Part model, mm, in its own coordinate system. Round coordinates to 2 decimals unless told otherwise and drop trailing zeros. Loops run counter-clockwise (first coordinate to the right, second up) from the corner with the lowest first, then second, coordinate; pieces in that order, holes last.
1) Drop flat-ended pins along their axis: P1, Ø3, axis at y = 1, z = -128.5, coming from the +X side; P2, Ø1.5, axis at x = 81.5, y = 2.5, coming from the +Z side; P3, Ø1, axis at x = -37, y = 4, coming from the -Z side. Give the stop position or say it passes through.
2) Band-saw the part on A-A, the plane x = 31. Write the cut outline in (y, z).
3) Probe line 1 (X direction, y = 3, z = -80); line 2 (Z direction, x = -93, y = 2.85); line 3 (Z direction, x = 26.5, y = 0.7). List the from-to ranges inside material, lowest first.
4) Band-saw the part on B-B, the plane y = 3.45. State how many separate pieces and enclosed holes the cut face has, then the cut area to 3 significant figures.
5) Band-saw the part on C-C, the plane x = -88.5. Write the cut outline in (y, z), then the cut area to 4 significant figures.
from build123d import *

# Parameters (mm, degrees)
SKETCH_1_W           = 213
SKETCH_1_H           = 190
EXTRUDE_1_DEPTH      = 5
SKETCH_2_R           = 2
SKETCH_2_R_2         = 6
CUT_EXTRUDE_1_DEPTH  = 143.801435567
SKETCH_3_W           = 213
SKETCH_3_H           = 5.445794932
CUT_EXTRUDE_2_DEPTH  = 143.801435567
SKETCH_4_W           = 28
SKETCH_4_H           = 35
CUT_EXTRUDE_3_DEPTH  = 143.801435567
FILLET_1_R           = 5
SKETCH_5_W           = 42
SKETCH_5_H           = 73.445794932
EXTRUDE_2_DEPTH      = 5
FILLET_2_R           = 20
SKETCH_6_R           = 2
CUT_EXTRUDE_4_DEPTH  = 200.352039946
SKETCH_7_R           = 2
CUT_EXTRUDE_5_DEPTH  = 200.352039946
SKETCH_8_W           = 20
SKETCH_8_H           = 22
SKETCH_8_H_2         = 28
CUT_EXTRUDE_6_DEPTH  = 200.352039946
FILLET_3_R           = 3
SKETCH_9_W           = 18
SKETCH_9_H           = 22
CUT_EXTRUDE_7_DEPTH  = 200.352039946
SKETCH_10_R          = 1.5
CUT_EXTRUDE_8_DEPTH  = 200.352039946
FILLET_4_R           = 10
SKETCH_11_W          = 115
SKETCH_11_H          = 70
CUT_EXTRUDE_9_DEPTH  = 200.352039946
FILLET_5_R           = 10
SKETCH_12_W          = 19.993467056
SKETCH_12_H          = 162.554205068
CUT_EXTRUDE_10_DEPTH = 200.352039946
FILLET_6_R           = 3
FILLET_7_R           = 10


with BuildPart() as part:
    # 草图1 → 凸台-拉伸1 (new body)
    with BuildSketch(Plane(origin=(0, 0, 0), x_dir=(1, 0, 0), z_dir=(0, 1, 0))):
        Rectangle(SKETCH_1_W, SKETCH_1_H)
    extrude(amount=EXTRUDE_1_DEPTH)

    # 草图2 → 切除-拉伸1 (cut, through all)
    with BuildSketch(Plane(origin=(0, 5, 0), x_dir=(1, 0, 0), z_dir=(0, 1, 0))):
        with Locations(Location((-9.5, 80, 0), (0, 0, 270))):
            Circle(SKETCH_2_R)
        with Locations(Location((46.5, 80, 0), (0, 0, 270))):
            Circle(SKETCH_2_R)
        with Locations(Location((-9.5, 50, 0), (0, 0, 270))):
            Circle(SKETCH_2_R)
        with Locations(Location((46.5, 50, 0), (0, 0, 270))):
            Circle(SKETCH_2_R)
        with Locations(Location((-39, -44.554205068, 0), (0, 0, 270))):
            Circle(SKETCH_2_R)
        with Locations(Location((17, -44.554205068, 0), (0, 0, 270))):
            Circle(SKETCH_2_R)
        with Locations(Location((17, -74.554205068, 0), (0, 0, 270))):
            Circle(SKETCH_2_R)
        with Locations(Location((-39, -74.554205068, 0), (0, 0, 270))):
            Circle(SKETCH_2_R)
        with Locations(Location((-11, -59.554205068, 0), (0, 0, 270))):
            Circle(SKETCH_2_R_2)
        with Locations(Location((18.5, 65, 0), (0, 0, 270))):
            Circle(SKETCH_2_R_2)
    extrude(amount=-CUT_EXTRUDE_1_DEPTH, mode=Mode.SUBTRACT)

    # 草图3 → 切除-拉伸2 (cut, through all)
    with BuildSketch(Plane(origin=(0, 5, 0), x_dir=(1, 0, 0), z_dir=(0, 1, 0))):
        with Locations((0, -92.277102534)):
            Rectangle(SKETCH_3_W, SKETCH_3_H)
    extrude(amount=-CUT_EXTRUDE_2_DEPTH, mode=Mode.SUBTRACT)

    # 草图4 → 切除-拉伸3 (cut, through all)
    with BuildSketch(Plane(origin=(0, 5, 0), x_dir=(1, 0, 0), z_dir=(0, 1, 0))):
        with Locations((-92.5, 1.945794932)):
            Rectangle(SKETCH_4_W, SKETCH_4_H)
    extrude(amount=-CUT_EXTRUDE_3_DEPTH, mode=Mode.SUBTRACT)

    # 圆角1
    fillet_1_edges = [part.edges().sort_by_distance(p)[0] for p in [
        (-106.5, 2.5, 15.554205068),
        (-106.5, 2.5, -19.445794932),
        (-78.5, 2.5, -19.445794932),
        (-78.5, 2.5, 15.554205068),
    ]]
    fillet(fillet_1_edges, radius=FILLET_1_R)

    # 草图5 → 凸台-拉伸2 (add)
    with BuildSketch(Plane(origin=(0, 5, 0), x_dir=(1, 0, 0), z_dir=(0, 1, 0))):
        with Locations((-85.5, 131.722897466)):
            Rectangle(SKETCH_5_W, SKETCH_5_H)
    extrude(amount=-EXTRUDE_2_DEPTH)

    # 圆角2
    fillet_2_edges = [part.edges().sort_by_distance(p)[0] for p in [
        (-64.5, 2.5, -95),
    ]]
    fillet(fillet_2_edges, radius=FILLET_2_R)

    # 草图6 → 切除-拉伸4 (cut, through all)
    with BuildSketch(Plane(origin=(0, 5, 0), x_dir=(1, 0, 0), z_dir=(0, 1, 0))):
        with Locations(Location((-96.5, 156.445794932, 0), (0, 0, 270))):
            Circle(SKETCH_6_R)
        with Locations(Location((-71.5, 156.445794932, 0), (0, 0, 270))):
            Circle(SKETCH_6_R)
        with Locations(Location((-71.5, 61.445794932, 0), (0, 0, 270))):
            Circle(SKETCH_6_R)
        with Locations(Location((-96.5, 61.445794932, 0), (0, 0, 270))):
            Circle(SKETCH_6_R)
    extrude(amount=-CUT_EXTRUDE_4_DEPTH, mode=Mode.SUBTRACT)

    # 草图7 → 切除-拉伸5 (cut, through all)
    with BuildSketch(Plane(origin=(0, 5, 0), x_dir=(1, 0, 0), z_dir=(0, 1, 0))):
        with Locations(Location((-96.5, 108.945794932, 0), (0, 0, 270))):
            Circle(SKETCH_7_R)
        with Locations(Location((-96.5, -24.554205068, 0), (0, 0, 270))):
            Circle(SKETCH_7_R)
        with Locations(Location((-96.5, -79.554205068, 0), (0, 0, 270))):
            Circle(SKETCH_7_R)
        with Locations(Location((81.5, 86.945794932, 0), (0, 0, 270))):
            Circle(SKETCH_7_R)
        with Locations(Location((81.5, 34.945794932, 0), (0, 0, 270))):
            Circle(SKETCH_7_R)
        with Locations(Location((81.5, -54.554205068, 0), (0, 0, 270))):
            Circle(SKETCH_7_R)
    extrude(amount=-CUT_EXTRUDE_5_DEPTH, mode=Mode.SUBTRACT)

    # 草图8 → 切除-拉伸6 (cut, through all)
    with BuildSketch(Plane(origin=(0, 5, 0), x_dir=(1, 0, 0), z_dir=(0, 1, 0))):
        with Locations((81.5, -78.554205068)):
            Rectangle(SKETCH_8_W, SKETCH_8_H)
        with Locations((81.5, -22.054205068)):
            Rectangle(SKETCH_8_W, SKETCH_8_H_2)
    extrude(amount=-CUT_EXTRUDE_6_DEPTH, mode=Mode.SUBTRACT)

    # 圆角3
    fillet_3_edges = [part.edges().sort_by_distance(p)[0] for p in [
        (91.5, 2.5, 89.554205068),
        (71.5, 2.5, 89.554205068),
        (71.5, 2.5, 67.554205068),
        (91.5, 2.5, 67.554205068),
        (71.5, 2.5, 36.054205068),
        (71.5, 2.5, 8.054205068),
    ]]
    fillet(fillet_3_edges, radius=FILLET_3_R)

    # 草图9 → 切除-拉伸7 (cut, through all)
    with BuildSketch(Plane(origin=(0, 5, 0), x_dir=(1, 0, 0), z_dir=(0, 1, 0))):
        with Locations((97.5, -78.554205068)):
            Rectangle(SKETCH_9_W, SKETCH_9_H)
    extrude(amount=-CUT_EXTRUDE_7_DEPTH, mode=Mode.SUBTRACT)

    # 草图10 → 切除-拉伸8 (cut, through all)
    with BuildSketch(Plane(origin=(0, 5, 0), x_dir=(1, 0, 0), z_dir=(0, 1, 0))):
        with Locations(Location((-83.5, 26.445794932, 0), (0, 0, 270))):
            Circle(SKETCH_10_R)
        with Locations(Location((-83.5, -22.554205068, 0), (0, 0, 270))):
            Circle(SKETCH_10_R)
    extrude(amount=-CUT_EXTRUDE_8_DEPTH, mode=Mode.SUBTRACT)

    # 圆角4
    fillet_4_edges = [part.edges().sort_by_distance(p)[0] for p in [
        (-106.5, 2.5, -168.445794932),
        (-64.5, 2.5, -168.445794932),
        (106.5, 2.5, 67.554205068),
        (-106.5, 2.5, 89.554205068),
        (106.5, 2.5, -95),
    ]]
    fillet(fillet_4_edges, radius=FILLET_4_R)

    # 草图11 → 切除-拉伸9 (cut, through all)
    with BuildSketch(Plane(origin=(0, 5, 0), x_dir=(1, 0, 0), z_dir=(0, 1, 0))):
        with Locations((1, 0.445794932)):
            Rectangle(SKETCH_11_W, SKETCH_11_H)
    extrude(amount=-CUT_EXTRUDE_9_DEPTH, mode=Mode.SUBTRACT)

    # 圆角5
    fillet_5_edges = [part.edges().sort_by_distance(p)[0] for p in [
        (-56.5, 2.5, 34.554205068),
        (-56.5, 2.5, -35.445794932),
        (58.5, 2.5, -35.445794932),
        (58.5, 2.5, 34.554205068),
    ]]
    fillet(fillet_5_edges, radius=FILLET_5_R)

    # 草图12 → 切除-拉伸10 (cut, through all)
    with BuildSketch(Plane(origin=(0, 5, 0), x_dir=(1, 0, 0), z_dir=(0, 1, 0))):
        with Locations((101.496733528, 13.722897466)):
            Rectangle(SKETCH_12_W, SKETCH_12_H)
    extrude(amount=-CUT_EXTRUDE_10_DEPTH, mode=Mode.SUBTRACT)

    # 圆角6
    fillet_6_edges = [part.edges().sort_by_distance(p)[0] for p in [
        (91.5, 2.5, 36.054205068),
        (91.5, 2.5, 8.054205068),
        (91.5, 2.5, 67.554205068),
    ]]
    fillet(fillet_6_edges, radius=FILLET_6_R)

    # 圆角7
    fillet_7_edges = [part.edges().sort_by_distance(p)[0] for p in [
        (91.5, 2.5, -95),
    ]]
    fillet(fillet_7_edges, radius=FILLET_7_R)


solid = part.part
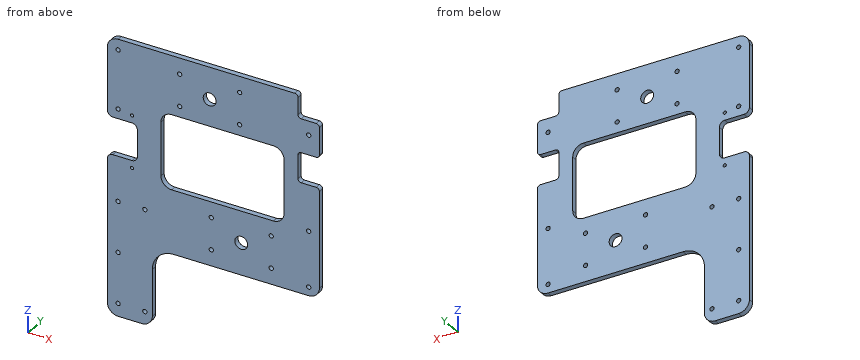
Reported:
1. P1: stops at x = -64.5
1. P2: stops at z = 67.55
1. P3: stops at z = -95
2. outline: (0, -95) - (5, -95) - (5, -35.45) - (0, -35.45) - close; (0, 34.55) - (5, 34.55) - (5, 89.55) - (0, 89.55) - close
3. line 1: x = -106.5 to -11.5, -7.5 to 44.5, 48.5 to 91.5
3. line 2: z = -168.45 to -19.45, 15.55 to 89.55
3. line 3: z = -95 to -35.45, 34.55 to 89.55
4. separate pieces: 1
4. enclosed holes: 23
4. area: 29,200 mm2
5. outline: (0, -168.45) - (5, -168.45) - (5, -19.45) - (0, -19.45) - close; (0, 15.55) - (5, 15.55) - (5, 89.55) - (0, 89.55) - close
5. area: 1,115 mm2
